Geometry check sheet. Reference: the model listing, model coordinates, mm. A direction names the side the tool comes from. Give positions to 0.01 mm unless a question says otherwise; leave off trailing zeros. Write each loop counter-clockwise with the first axis right and the second up, starting at its lowest first coordinate (ties: lowest second). Pieces come first, ordered by that corner, then holes. Notation, with made-up numbers: (87.25, 76) - (135.25, 76) arc R20 cw to (135.25, 106) - close; hole circle Ø4 at (41.25, -2). An arc over 180 degrees is marked (long way). Use a Markdown table: item, result.
```python
from build123d import *

# Parameters (mm, degrees)
BASE_FLANGE1_DEPTH      = 25
CUT_EXTRUDE1_DEPTH      = 38.336309405
CUT_EXTRUDE1_DEPTH_BACK = 38.336309405
SKETCH6_W               = 21.5
SKETCH6_H               = 15
CUT_EXTRUDE2_DEPTH      = 38.336309405
CUT_EXTRUDE2_DEPTH_BACK = 38.336309405
SKETCH7_R               = 0.75
SKETCH7_W               = 1.5
SKETCH7_H               = 3.5
CUT_EXTRUDE3_DEPTH      = 38.027017163
CUT_EXTRUDE3_DEPTH_BACK = 38.027017163


# Sheet-metal steps are written as plain solids
with BuildPart() as part:
    # Sketch1 → Base-Flange1 (new body)
    with BuildSketch(Plane(origin=(0, 0, 0), x_dir=(0, 1, 0), z_dir=(0, 0, 1))):
        with BuildLine():
            Line((0, 0), (12, 0))
            ThreePointArc((12, 0), (13.414213562, -0.585786438), (14, -2))
            Line((14, -2), (14, -10))
            ThreePointArc((14, -10), (14.292893219, -10.707106781), (15, -11))
            Line((15, -11), (25, -11))
            Line((25, -11), (25, -12))
            Line((25, -12), (15, -12))
            ThreePointArc((15, -12), (13.585786438, -11.414213562), (13, -10))
            Line((13, -10), (13, -2))
            ThreePointArc((13, -2), (12.707106781, -1.292893219), (12, -1))
            Line((12, -1), (0, -1))
            Line((0, -1), (0, 0))
        make_face()
    extrude(amount=BASE_FLANGE1_DEPTH)

    # Sketch6 → Cut-Extrude1 (cut, two sides: drawn at the far end of the back side and taken through both)
    with BuildSketch(Plane.YZ.offset(-CUT_EXTRUDE1_DEPTH_BACK)):
        with Locations((10.75, 17.5)):
            Rectangle(SKETCH6_W, SKETCH6_H)
    extrude(amount=CUT_EXTRUDE1_DEPTH + CUT_EXTRUDE1_DEPTH_BACK, mode=Mode.SUBTRACT)

    # Sketch7 → Cut-Extrude2 (cut, two sides: drawn at the far end of the back side and taken through both)
    with BuildSketch(Plane.YZ.offset(12).offset(-CUT_EXTRUDE2_DEPTH_BACK)):
        with Locations(Location((23.25, 22, 0), (0, 0, 90))):
            Circle(SKETCH7_R)
        with Locations(Location((23.25, 18, 0), (0, 0, 90))):
            Circle(SKETCH7_R)
        with Locations((23.25, 13.25)):
            Rectangle(SKETCH7_W, SKETCH7_H)
    extrude(amount=CUT_EXTRUDE2_DEPTH + CUT_EXTRUDE2_DEPTH_BACK, mode=Mode.SUBTRACT)

    # Sketch8 → Cut-Extrude3 (cut, two sides: drawn at the far end of the back side and taken through both)
    with BuildSketch(Plane.YZ.offset(1).offset(-CUT_EXTRUDE3_DEPTH_BACK)):
        Polygon((2.577350269, 5), (2.288675135, 5.5), (1.711324865, 5.5), (1.422649731, 5), (1.711324865, 4.5), (2.288675135, 4.5), align=None)
        Polygon((6.732050808, 5), (6.443375673, 5.5), (5.866025404, 5.5), (5.577350269, 5), (5.866025404, 4.5), (6.443375673, 4.5), align=None)
    extrude(amount=CUT_EXTRUDE3_DEPTH + CUT_EXTRUDE3_DEPTH_BACK, mode=Mode.SUBTRACT)


solid = part.part
```
1) Mould release check, pull along Z, two halves, no side actions. Record for faces 1 (the cylindrical face through (11.493, 23.982, 17.837)), 2 (the cylindrical face through (0.57, 13.4, 4.93)), 3 (the flat face through (5.5, 13.5, 0)), 4 (the flat face through (11.5, 23.2, 11.5)): pulls with the +Z half, pulls with the -Z half, needs draft (parallel to the pull), parting line crosses it, or undercut.
Working result:
| item | result |
|---|---|
| face 1 | undercut |
| face 2 | needs draft |
| face 3 | pulls with the -Z half |
| face 4 | undercut |
2) Section check B-B on z = 22. Record the boundary of the cut face in (x, y).
Working result:
| item | result |
|---|---|
| outline | (11, 21.5) - (12, 21.5) - (12, 22.5) - (11, 22.5) - close; (11, 24) - (12, 24) - (12, 25) - (11, 25) - close |
3) Material ranges on L1, parallel to Y at x = 11.4, z = 22; L2, parallel to Z at x = 1.25, y = 13.5; L3, parallel to Y at x = 8.75, z = 5, recorded low to high. Write a range as from..to.
Working result:
| item | result |
|---|---|
| L1 | y = 21.5..22.5, 24..25 |
| L2 | z = 0..10 |
| L3 | y = 13..14 |
4) Section check A-A on y = 23.25. Record the boundary of the cut face in (x, z).
Working result:
| item | result |
|---|---|
| outline | (11, 0) - (12, 0) - (12, 11.5) - (11, 11.5) - close; (11, 15) - (12, 15) - (12, 17.25) - (11, 17.25) - close; (11, 18.75) - (12, 18.75) - (12, 21.25) - (11, 21.25) - close; (11, 22.75) - (12, 22.75) - (12, 25) - (11, 25) - close |
5) Section check D-D on x = 7. Record the boundary of the cut face in (y, z).
Working result:
| item | result |
|---|---|
| outline | (13, 0) - (14, 0) - (14, 10) - (13, 10) - close |
6) Set-up check for faces 5 (the flat face through (11, 21, 9.5)), 6 (the flat face through (6, 13, 5)), 7 (the flat face through (11.5, 21.5, 17.4)): record each of +Z, -Z, +X, -X, +Y, -Y from which the full face is reachable in a straight line by a thin tool's end or side.
Working result:
| item | result |
|---|---|
| face 5 | +Z, -Z, -X, +Y |
| face 6 | +Z, -Z, +X, -Y |
| face 7 | +Z, +X, -X, -Y |
7) Depth check by flat-ended pin: P1, Ø1.1, axis at x = 11.5, z = 16, coming from the -Y side; P2, Ø5, axis at y = 4.5, z = 5, coming from the +X side; P3, Ø1.4, axis at y = 23.25, z = 22, coming from the +X side; P4, Ø3, axis at y = 20.5, z = 18, coming from the -X side. Enter the tip coordinate at first touch or a pass-through.
Working result:
| item | result |
|---|---|
| P1 | stops at y = 21.5 |
| P2 | stops at x = 1 |
| P3 | passes through |
| P4 | stops at x = 11 |
8) Section check C-C on z = 4. Record the boundary of the cut face in (x, y), then the cut area to 3 significant figures.
Working result:
| item | result |
|---|---|
| outline | (0, 0) - (1, 0) - (1, 12) arc R1 cw to (2, 13) - (10, 13) arc R2 ccw to (12, 15) - (12, 25) - (11, 25) - (11, 15) arc R1 cw to (10, 14) - (2, 14) arc R2 ccw to (0, 12) - close |
| area | 34.7 mm² |
